Build history of the part. All positions in model axes, mm. A direction names the side the tool comes from. Give positions to 0.01 mm unless a question says otherwise; leave off trailing zeros. Order: outer loops, then holes, each group sorted by start corner. A loop starts at its lowest first (then second) coordinate and runs counter-clockwise, first axis right, second up. Notation, with made-up numbers: (-6.75, 44) - (52.25, 44) arc R28 cw to (52.25, 75) - close; hole circle Ø5 at (29.5, 89). An arc over 180 degrees is marked (long way). One line per item, written item: value.
```python
from build123d import *

# Parameters (mm, degrees)
F0_R      = 7
F0_R_2    = 5.5
F1_DEPTH  = 44
F2_W      = 20
F2_H      = 19
F2_W_2    = 7
F3_DEPTH  = 51.001
F6_DEPTH  = 24
F8_DEPTH  = 19
F9_R      = 5.5
F10_DEPTH = 7
F11_DEPTH = 32


with BuildPart() as f1:
    # F0 (on Front) → F1 (new body)
    with BuildSketch(Plane.XZ):
        with BuildLine():
            Line((-5, 24), (-29, 24))
            ThreePointArc((-29, 24), (-37.4389012943, 14.9820441422), (-49.6386191642, 13.0570852328))
            Line((-49.6386191642, 13.0570852328), (-72, 17))
            Line((-72, 17), (-79, 17))
            Line((-79, 17), (-86, 10))
            Line((-86, 10), (-86, -8))
            Line((-86, -8), (-79, -15))
            Line((-79, -15), (-46.4244610887, -15))
            ThreePointArc((-46.4244610887, -15), (-43.1592253076, -16.2134137678), (-41.4788223472, -19.2647058824))
            ThreePointArc((-41.4788223472, -19.2647058824), (-39.1419921441, -27.115672061), (-34.7030199473, -34))
            Line((-34.7030199473, -34), (-29, -34))
            Line((-29, -34), (0, 0))
            Line((0, 0), (0, 19))
            Line((0, 19), (-5, 24))
        make_face()
        with Locations((-72, -1)):
            Circle(F0_R, mode=Mode.SUBTRACT)
        with Locations((-14, 10)):
            Circle(F0_R_2, mode=Mode.SUBTRACT)
    extrude(amount=F1_DEPTH)

    # F2 (on face) → F3 (cut, through all)
    with BuildSketch(Plane.XY.offset(17)):
        with Locations((-62, -34.5)):
            Rectangle(F2_W, F2_H)
        with Locations((-75.5, -34.5)):
            Rectangle(F2_W_2, F2_H)
        with Locations((-82.5, -34.5)):
            Rectangle(F2_W_2, F2_H)
    extrude(amount=-F3_DEPTH, mode=Mode.SUBTRACT)

    # F5 (on offset) → F6 (cut)
    with BuildSketch(Plane.XZ.offset(12)):
        with BuildLine():
            Line((-10.2352941176, -12), (0, 0))
            Line((0, 0), (0, 19))
            Line((0, 19), (-5, 24))
            Line((-5, 24), (-29, 24))
            ThreePointArc((-29, 24), (-32.9787556567, 18.2593336205), (-38.763063451, 14.3442946173))
            ThreePointArc((-38.763063451, 14.3442946173), (-27.8157370175, -2.4192947713), (-10.2352941176, -12))
        make_face()
    extrude(amount=F6_DEPTH, mode=Mode.SUBTRACT)

    # F7 (on face) → F8 (cut)
    with BuildSketch(Plane.XZ.offset(44)):
        with BuildLine():
            Line((-46.4244610887, -15), (-52, -15))
            Line((-52, -15), (-52, -51.1183999479))
            Line((-52, -51.1183999479), (24.7316434979, -51.1183999479))
            Line((24.7316434979, -51.1183999479), (24.7316434979, -15))
            Line((24.7316434979, -15), (-12.7941176471, -15))
            Line((-12.7941176471, -15), (-29, -34))
            Line((-29, -34), (-34.7030199473, -34))
            ThreePointArc((-34.7030199473, -34), (-39.1419921441, -27.115672061), (-41.4788223472, -19.2647058824))
            ThreePointArc((-41.4788223472, -19.2647058824), (-43.1592253076, -16.2134137678), (-46.4244610887, -15))
        make_face()
        with BuildLine():
            Line((-12.7941176471, -15), (-46.4244610887, -15))
            ThreePointArc((-46.4244610887, -15), (-43.1592253076, -16.2134137678), (-41.4788223472, -19.2647058824))
            ThreePointArc((-41.4788223472, -19.2647058824), (-39.1419921441, -27.115672061), (-34.7030199473, -34))
            Line((-34.7030199473, -34), (-29, -34))
            Line((-29, -34), (-12.7941176471, -15))
        make_face()
    extrude(amount=-F8_DEPTH, mode=Mode.SUBTRACT)

    # F9 (on face) → F10 (cut)
    with BuildSketch(Plane.XZ.offset(44)):
        with BuildLine():
            ThreePointArc((-28.3639153145, 23), (-32.8995598011, 16.9571773079), (-39.3533170567, 13.0282087051))
            ThreePointArc((-39.3533170567, 13.0282087051), (-28.689818317, -2.9721273618), (-12.0131522532, -12.5434265746))
            Line((-12.0131522532, -12.5434265746), (-1, 0.3685450325))
            Line((-1, 0.3685450325), (-1, 18.5857864376))
            Line((-1, 18.5857864376), (-5.4142135624, 23))
            Line((-5.4142135624, 23), (-28.3639153145, 23))
        make_face()
        with Locations((-14, 10)):
            Circle(F9_R, mode=Mode.SUBTRACT)
    extrude(amount=-F10_DEPTH, mode=Mode.SUBTRACT)

    # F9 (on face) → F11 (cut, through all)
    with BuildSketch(Plane.XZ.offset(44)):
        with BuildLine():
            Line((-51, 12.3190646627), (-51, -14))
            Line((-51, -14), (-13.2555237042, -14))
            Line((-13.2555237042, -14), (-12.0131522532, -12.5434265746))
            ThreePointArc((-12.0131522532, -12.5434265746), (-28.689818317, -2.9721273618), (-39.3533170567, 13.0282087051))
            ThreePointArc((-39.3533170567, 13.0282087051), (-45.1237934763, 11.805403344), (-51, 12.3190646627))
        make_face()
    extrude(amount=-F11_DEPTH, mode=Mode.SUBTRACT)


solid = f1.part
```
(1) Pull direction X, two halves, no side cores. Call faces 5 (the face through (-75, -12, 17)), 6 (the face through (-51, -28, -1)), 7 (the face through (-28.02, -23.83, -2.23)): +X half, -X half, draft (parallel to the pull), parting line (faces both ways), or undercut.
Completed:
face 5: draft
face 6: undercut
face 7: +X half
(2) Slice it at D-D, the plane z = -1. Give the cut face in (x, y), and give its area (3 significant figures).
Completed:
outline: (-86, -25) - (-79, -25) - (-79, 0) - (-86, 0) - close; (-65, -25) - (-52, -25) - (-52, -44) - (-51, -44) - (-51, -12) - (-30.66, -12) - (-30.66, -37) - (-2.17, -37) - (-2.17, -44) - (-0.85, -44) - (-0.85, -36) - (-29.28, -36) - (-29.28, -12) - (-0.85, -12) - (-0.85, 0) - (-65, 0) - close
area: 1,220 mm²
(3) Drill centre lines: line 1 (X direction, y = -36.4, z = 10); line 2 (Z direction, x = -14, y = -36.7); line 3 (X direction, y = -17, z = -1). Where is each one in solid material? Low to high.
Completed:
line 1: -52 to -51, -38.09 to -19.5, -8.5 to 0
line 2: -15 to -14, -11.9 to 4.5, 15.5 to 24
line 3: -86 to -79, -65 to -51, -30.66 to -29.28
(4) Slice it at A-A, the plane y = -27. Give the cut face in (x, z).
Completed:
outline: (-52, -15) - (-12.79, -15) - (-10.24, -12) arc R41 cw to (-38.76, 14.34) arc R19 cw to (-49.64, 13.06) - (-52, 13.47) - close; hole (-51, -14) - (-13.26, -14) - (-12.01, -12.54) arc R42 cw to (-39.35, 13.03) arc R20 cw to (-51, 12.32) - close
(5) Slice it at B-B, the plane y = -10. Give the cut face in (x, z), and give its area (3 significant figures).
Completed:
outline: (-86, -8) - (-79, -15) - (-46.42, -15) arc R5 cw to (-41.48, -19.26) arc R29 ccw to (-34.7, -34) - (-29, -34) - (0, 0) - (0, 19) - (-5, 24) - (-29, 24) arc R19 cw to (-49.64, 13.06) - (-72, 17) - (-79, 17) - (-86, 10) - close; hole circle Ø14 at (-72, -1); hole circle Ø11 at (-14, 10)
area: 2,830 mm²
(6) Pin check, flat tips, straight feed: P1, Ø11, axis at x = -13.5, z = -2, coming from the +Y side; P2, Ø15, axis at y = -35, z = -6.5, coming from the -X side; P3, Ø13.5, axis at x = -29, z = -6, coming from the -Y side; P4, Ø9.5, axis at x = -23.5, z = -26, coming from the -Y side. Stop position of each tip, or through.
Completed:
P1: y = 0
P2: x = -52
P3: y = -37
P4: y = -25
(7) 3-axis set-ups, long thin cutter, end or side, ignore diameter. For faces 1 (the face through (-2, -40, 21)), 2 (the face through (-20, -36, 10)), 3 (the face through (-20, -37, 5)), 4 (the face through (-46, -27, -15)): which of +Z, -Z, +X, -X, +Y, -Y reach the whole face in a straight line?
Completed:
face 1: +Z, +X, +Y, -Y
face 2: +Z, +X
face 3: -Y
face 4: -Z, -X, -Y
(8) Slice it at C-C, the plane z = 7. Give the cut face in (x, y).
Completed:
outline: (-86, -25) - (-52, -25) - (-52, -44) - (-51, -44) - (-51, -12) - (-36.54, -12) - (-36.54, -37) - (-18.61, -37) - (-18.61, -36) - (-35.39, -36) - (-35.39, -12) - (-18.61, -12) - (-18.61, 0) - (-86, 0) - close; (-9.39, -37) - (-1, -37) - (-1, -44) - (0, -44) - (0, -36) - (-9.39, -36) - close; (-9.39, -12) - (0, -12) - (0, 0) - (-9.39, 0) - close
